```python
from build123d import *

# Parameters (mm, degrees)
SKETCH1_R           = 1.55
SKETCH1_R_2         = 1.5
SKETCH1_R_3         = 3.5
SKETCH1_W           = 5
SKETCH1_H           = 4
SKETCH1_W_2         = 5.253269852
SKETCH1_H_2         = 20.055
BOSS_EXTRUDE1_DEPTH = 4


with BuildPart() as part:
    # Sketch1 → Boss-Extrude1 (new body)
    with BuildSketch(Plane(origin=(0, 0, 0), x_dir=(1, 0, 0), z_dir=(0, 1, 0))):
        with BuildLine():
            Line((-58, -40), (58, -40))
            ThreePointArc((58, -40), (62.949747468, -37.949747468), (65, -33))
            Line((65, -33), (65, 33))
            ThreePointArc((65, 33), (62.949747468, 37.949747468), (58, 40))
            Line((58, 40), (-58, 40))
            ThreePointArc((-58, 40), (-62.949747468, 37.949747468), (-65, 33))
            Line((-65, 33), (-65, -33))
            ThreePointArc((-65, -33), (-62.949747468, -37.949747468), (-58, -40))
        make_face()
        with Locations(Location((61, 25.5, 0), (0, 0, 270))):
            Circle(SKETCH1_R, mode=Mode.SUBTRACT)
        with Locations(Location((61, -25.5, 0), (0, 0, 90))):
            Circle(SKETCH1_R, mode=Mode.SUBTRACT)
        with Locations(Location((-61, -25.5, 0), (0, 0, 270))):
            Circle(SKETCH1_R, mode=Mode.SUBTRACT)
        with Locations(Location((-61, 25.5, 0), (0, 0, 90))):
            Circle(SKETCH1_R, mode=Mode.SUBTRACT)
        with Locations(Location((-5.1, -7.2275, 0), (0, 0, 270))):
            Circle(SKETCH1_R_2, mode=Mode.SUBTRACT)
        with Locations(Location((-5.1, 7.2275, 0), (0, 0, 270))):
            Circle(SKETCH1_R_2, mode=Mode.SUBTRACT)
        with Locations(Location((35, 0, 0), (0, 0, 270))):
            Circle(SKETCH1_R_3, mode=Mode.SUBTRACT)
        with Locations((58.5, 18.5)):
            Rectangle(SKETCH1_W, SKETCH1_H, mode=Mode.SUBTRACT)
        with Locations((58.5, -18.5)):
            Rectangle(SKETCH1_W, SKETCH1_H, mode=Mode.SUBTRACT)
        with Locations((-58.5, -18.5)):
            Rectangle(SKETCH1_W, SKETCH1_H, mode=Mode.SUBTRACT)
        with Locations((-58.5, 18.5)):
            Rectangle(SKETCH1_W, SKETCH1_H, mode=Mode.SUBTRACT)
        with Locations((5.848955237, 0)):
            Rectangle(SKETCH1_W_2, SKETCH1_H_2, mode=Mode.SUBTRACT)
    extrude(amount=BOSS_EXTRUDE1_DEPTH)


solid = part.part
```
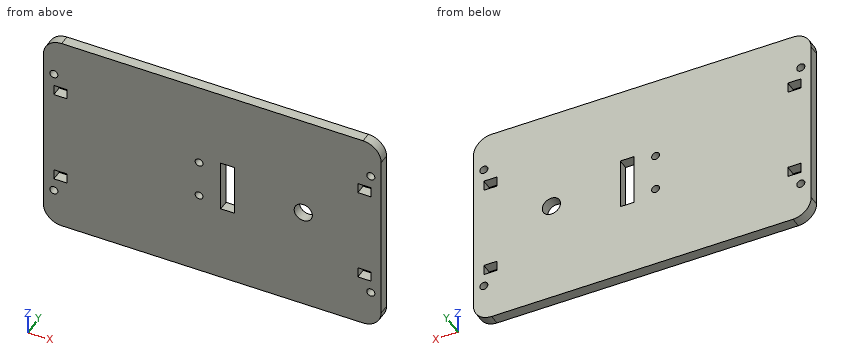
Here's how the part is built. I have some questions about the finished solid (model axes, mm). Coordinates: 2 decimals unless noted, no trailing zeros. Order: outer loops, then holes, each group sorted by start corner. A loop starts at its lowest first (then second) coordinate and runs counter-clockwise, first axis right, second up. Notation, with made-up numbers: M 53.5,-2 L 108.5,-2 A22 cw 108.5,22 Z; hole C 14.25,-32.5 d2. An arc over 180 degrees is marked long. Answer as a JSON object with one key per item and string values. Group by question number.
(1) Suppose I cut it at C-C, the plane y = 1.6. State how many separate pieces and enclosed holes the cut face has, then the cut area to 3 significant figures.
(2) For pin 1 (1.2 mm diameter, centred on x = -59.5, y = 2, fed in from +Z); pin 2 (2 mm diameter, centred on x = 59.5, y = 3, fed in from -Z), each with a flat end and sliding along its axis, tell me the tip position at first contact or that it passes through.
(3) I need wall thicknesses on probe 1 along Z at (x, y) = (-5, 1.8); probe 2 along X at (y, z) = (1.3, -25.5); probe 3 along X at (y, z) = (2.5, 0). Which ranges of each line are inside material? Lowest first, please.
(4) Suppose I cut it at B-B, the plane x = -5.1. Please give me the cut outline in (y, z).
(5) Suppose I cut it at A-A, the plane z = 0. Please give me the cut outline in (x, y), then the cut area to 3 significant figures.
Values found:
{
 "1": {"separate pieces": "1", "enclosed holes": "12", "area": "10,100 mm^2"},
 "2": {"pin 1": "stops at z = 39.94", "pin 2": "stops at z = -39.98"},
 "3": {"probe 1": "z = -40 to -8.72, -5.73 to 5.73, 8.72 to 40", "probe 2": "x = -65 to -62.55, -59.45 to 59.45, 62.55 to 65", "probe 3": "x = -65 to 3.22, 8.48 to 31.5, 38.5 to 65"},
 "4": {"outline": "M 0,-40 L 4,-40 L 4,-8.73 L 0,-8.73 Z; M 0,-5.73 L 4,-5.73 L 4,5.73 L 0,5.73 Z; M 0,8.73 L 4,8.73 L 4,40 L 0,40 Z"},
 "5": {"outline": "M -65,0 L 3.22,0 L 3.22,4 L -65,4 Z; M 8.48,0 L 31.5,0 L 31.5,4 L 8.48,4 Z; M 38.5,0 L 65,0 L 65,4 L 38.5,4 Z", "area": "471 mm^2"}
}
